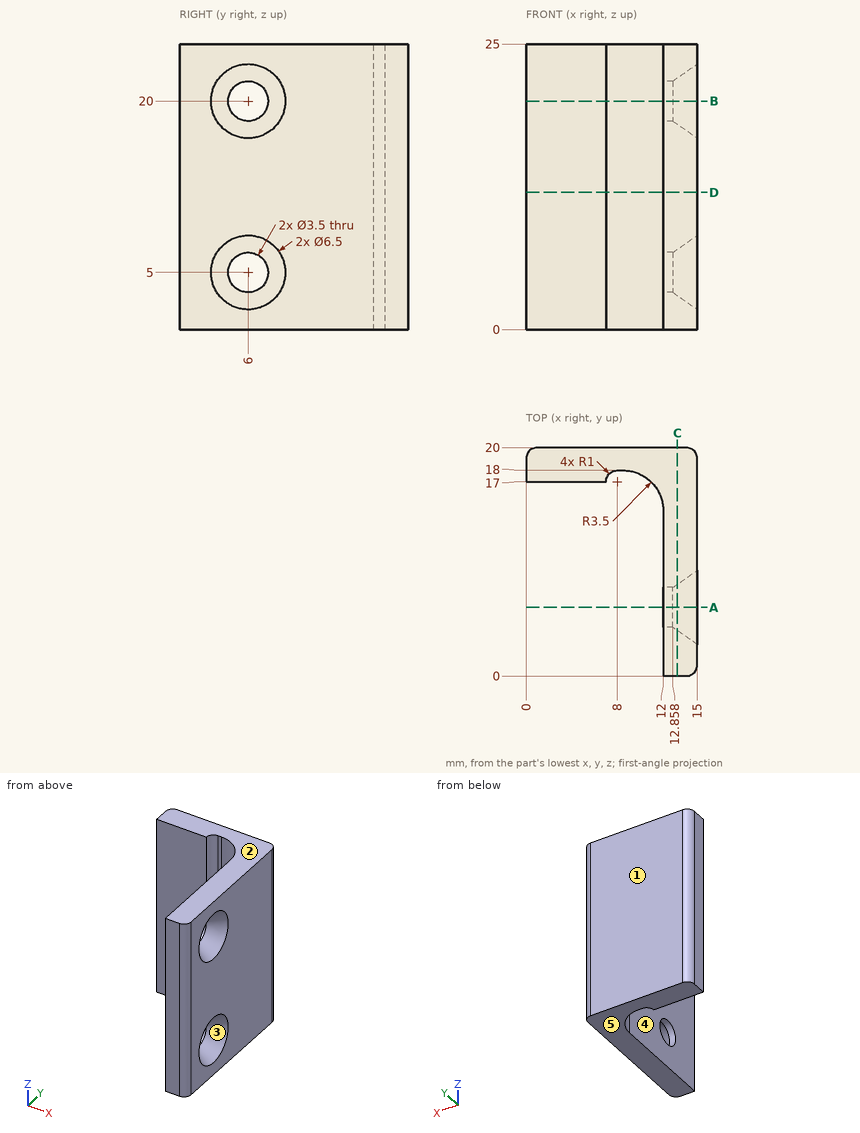
Geometry check sheet. Reference: drawing and pictorial views, mm from the part's lowest x, y, z. A direction names the side the tool comes from. Give positions to 0.01 mm unless a question says otherwise; leave off trailing zeros. Write each loop counter-clockwise with the first axis right and the second up, starting at its lowest first coordinate (ties: lowest second). Pieces come first, ordered by that corner, then holes. Notation, with made-up numbers: M -4.5,-19 L 39.5,-19 A31 ccw 39.5,15 Z; hole C 79,76 d3. An arc over 180 degrees is marked long. Use CSV: the item, a comma, the result in double quotes.
1) Cross-section at C-C (x = 13.25). Enter the section's corners in (y, z) (1 decimal), plus the area to 3 significant figures.
Final values:
outline,"M 0,0 L 20,0 L 20,25 L 0,25 Z; hole C 6,5 d4; hole C 6,20 d4"
area,"474 mm²"
2) Release check for a two-part mould opening along Y. For the marked faces 1, 2 and 3 record: released by +Y, released by -Y, zero draft, split by the parting line, or undercut.
Final values:
face 1,"released by +Y"
face 2,"zero draft"
face 3,"undercut"
3) Cross-section at D-D (z = 12). Enter the section's corners in (x, y).
Final values:
outline,"M 0,17 L 7,17 A1 cw 8,18 L 8.5,18 A3.5 cw 12,14.5 L 12,0 L 14,0 A1 ccw 15,1 L 15,19 A1 ccw 14,20 L 1,20 A1 ccw 0,19 Z"
4) Access from +Z, -Z, +X, -X, +Y, -Y to the whole of each face (thin tool, end or side, straight path). Record for the marked faces 4 and 5.
Final values:
face 4,"+Z, -Z, -X, -Y"
face 5,"-Z, +X, -X, +Y, -Y"
5) Cross-section at A-A (y = 6). Enter the section's corners in (x, z).
Final values:
outline,"M 12,0 L 15,0 L 15,1.75 L 12.86,3.25 L 12,3.25 Z; M 12,6.75 L 12.86,6.75 L 15,8.25 L 15,16.75 L 12.86,18.25 L 12,18.25 Z; M 12,21.75 L 12.86,21.75 L 15,23.25 L 15,25 L 12,25 Z"
6) Material ranges on line 1 along Z through (x, y) = (12.2, 6); line 2 along Z through (x, y) = (13.75, 7.5); line 3 along Y through (x, z) = (12.65, 20), recorded low to high.
Final values:
line 1,"0 to 3.25, 6.75 to 18.25, 21.75 to 25"
line 2,"0 to 3.16, 6.84 to 18.16, 21.84 to 25"
line 3,"0 to 4.25, 7.75 to 20"
7) Cross-section at B-B (z = 20). Enter the section's corners in (x, y), plus the area to 3 significant figures.
Final values:
outline,"M 0,17 L 7,17 A1 cw 8,18 L 8.5,18 A3.5 cw 12,14.5 L 12,7.75 L 12.86,7.75 L 15,9.25 L 15,19 A1 ccw 14,20 L 1,20 A1 ccw 0,19 Z; M 12,0 L 14,0 A1 ccw 15,1 L 15,2.75 L 12.86,4.25 L 12,4.25 Z"
area,"79.5 mm²"
8) Go/stop test with flat-tipped pins: pin 1 Ø3 at (y, z) = (3.5, 7) entering from -X; pin 2 Ø2 at (x, z) = (2.5, 11) entering from -Y. Record where each tip stops, or that it passes through.
Final values:
pin 1,"x = 12"
pin 2,"y = 17"
